Autodesk Inventor part; units mm, degrees
ref_plane "Work Plane1" through (0, 0, 2) normal (0, 0, -1) x (-1, 0, 0)
ref_plane "Work Plane2" through (0, 0, 15.2) normal (0, 0, -1) x (-1, 0, 0)
ref_plane "YZ Plane" through (0, 0, 0) normal (1, 0, 0) x (0, 1, 0)
sketch "Sketch1" plane through (0, 0, 0) normal (0, 0, 1) x (1, 0, 0)
  circle A0 centre (0, 0) radius 37.5 construction
  circle A1 centre (0, 0) radius 38.1
  line L0 (0, 0) -> (0, 82.8508) construction
  line L1 (-6, 47.5) -> (6, 47.5)
  line L2 (20, 35.8331) -> (20, 38.2923)
  line L3 (-20, 35.8331) -> (-20, 38.2923)
  arc A2 (-6, 47.5) -> (-18.8366, 41.4986) centre (-6, 30.7709) ccw
  arc A3 (18.8366, 41.4986) -> (6, 47.5) centre (6, 30.7709) ccw
  arc A4 (-18.8366, 41.4986) -> (-20, 38.2923) centre (-15, 38.2923) ccw
  arc A5 (20, 38.2923) -> (18.8366, 41.4986) centre (15, 38.2923) ccw
  arc A6 (17.1022, 34.0459) -> (-17.1022, 34.0459) centre (0, 0) ccw
  arc A7 (-20, 35.8331) -> (-17.1022, 34.0459) centre (-18, 35.8331) ccw
  arc A8 (17.1022, 34.0459) -> (20, 35.8331) centre (18, 35.8331) ccw
  point P0 (20, 32.4285)
  point P1 (20, 39.9285)
  point P2 (-20, 32.4285)
  point P3 (-20, 39.9285)
  point P4 (-17.1022, 34.0459)
  dimension "d0" = 75
  dimension "d1" = 0.6
  dimension "d22" = 12
  dimension "d23" = 6
  dimension "d24" = 47.5
  dimension "d25" = 7.5
  dimension "d26" = 7.5
  dimension "d27" = 40
  dimension "d28" = 20
  dimension "d29" = 5
  dimension "d30" = 2
extrude "Extrusion1" add sketch "Sketch1" along normal blind 30.4 contours A1 A7 L3 A4 A2 L1 A3 A5 L2 A8
sketch "Sketch2" plane through (-6, 47.5, 0) normal (0, 1, 0) x (1, 0, 0)
  line L0 (12, -30.4) -> (0, -30.4)
  line L1 (12, 0) -> (12, -30.4)
  line L2 (0, -30.4) -> (16.9706, -30.4) construction
  line L3 (12, -30.4) -> (24.8366, -30.4)
  line L4 (0, 0) -> (0, -30.4)
  line L5 (23.1022, 0) -> (-11.1022, 0)
  circle A0 centre (6, -22.4) radius 3.9
  circle A1 centre (6, -8) radius 3.9
  point P0 (6, 0)
  dimension "d34" = 7.8
  dimension "d35" = 7.8
  dimension "d38" = 12
  dimension "d39" = 6
  dimension "d40" = 6
  dimension "d41" = 8
  dimension "d42" = 8
extrude "Extrusion2" cut sketch "Sketch2" against normal blind 15 contours A0 | A1
ref_plane "Work Plane1" through (0, 0, 2) normal (0, 0, -1) x (-1, 0, 0)
sketch "Sketch3" plane through (0, 0, 2) normal (0, 0, -1) x (-1, 0, 0)
  arc A0 (17.1022, 34.0459) -> (-17.1022, 34.0459) centre (0, 0) ccw
  line L0 (-15, 35.023) -> (-15, 36.023)
  line L1 (15, 35.023) -> (15, 36.023)
  line L2 (0, 0) -> (0, 39.8883) construction
  arc A1 (15, 36.023) -> (-15, 36.023) centre (0, 0) ccw
  dimension "d44" = 1
  dimension "d45" = 30
  dimension "d46" = 15
extrude "Extrusion3" cut sketch "Sketch3" against normal blind 26.4
sketch "Sketch4" plane through (0, 0, 0) normal (0, 0, -1) x (-1, 0, 0)
  line L0 (-6, 47.5) -> (6, 47.5)
  circle A0 centre (-12, 41.5) radius 2.4
  line L1 (-6, 47.5) -> (6, 47.5)
  circle A1 centre (12, 41.5) radius 2.4
  point P0 (0, 0)
  dimension "d52" = 4.8
  dimension "d53" = 12
  dimension "d54" = 6
  dimension "d55" = 4.8
  dimension "d56" = 12
  dimension "d57" = 6
extrude "Extrusion4" cut sketch "Sketch4" against normal blind 8
ref_plane "Work Plane2" through (0, 0, 15.2) normal (0, 0, -1) x (-1, 0, 0)
mirror "Mirror1" about plane through (0, 0, 15.2) normal (0, 0, -1) of "Extrusion4"
equation "\"d23\" = 0.5 * d22"
equation "\"d35\" = d34"
equation "\"d39\" = 0.5 * d38"
equation "\"d40\" = 0.5 * d38"
equation "\"d42\" = d41"
equation "\"d46\" = 0.5 * d45"
equation "\"d57\" = d54"
properties part number "PipeHolder" material "ABS Plastic"
Can you work these out from the model? Positions are in its coordinate system, mm. A direction names the side the tool comes from. Round coordinates to 2 decimals unless told otherwise and drop trailing zeros. Loops run counter-clockwise (first coordinate to the right, second up) from the corner with the lowest first, then second, coordinate; pieces in that order, holes last. Notation, with made-up numbers: (-31, 50.5) - (-18, 50.5) arc R22 ccw to (-18, 78.5) - close; hole circle Ø6 at (19, 63.5). An arc over 180 degrees is marked (long way). Answer in a Markdown table with one row per item. Add a question column.
Q1. I need wall thicknesses on L1, parallel to X at y = 41.75, z = 24.5; L2, parallel to Z at x = 0.5, y = 38.25; L3, parallel to Y at x = 14, z = 27. Which ranges of each line are inside material? Lowest first, please.
Q2. I want a section at B-B on x = -2.5. List the corners of the cut face in (y, z) for me, and give its area (3 significant figures).
Q3. I want a section at C-C on z = 8.5. List the corners of the cut face in (x, y) for me.
Q4. I want a section at A-A on z = 3. List the corners of the cut face in (x, y) for me, and give its area (3 significant figures).
Q5. For pin 1 Ø2.5 at (x, y) = (-12, 41) entering from -Z; pin 2 Ø0.5 at (y, z) = (35.5, 16.5) entering from -X; pin 3 Ø3 at (y, z) = (44, 9) entering from +X; pin 4 Ø8 at (x, z) = (10.5, 25.5) entering from +Y, each with a flat end and sliding along its axis, tell me the tip position at first contact or that it passes through.
Q6. We'd pull the mould along Z, two halves only. Please class faces 1 (the flat face through (0, 41, 30.4)), 2 (the cylindrical face through (12.99, 45.97, 14.99)), 3 (the flat face through (0.1, 38.5, 2)): pulls with the +Z half, pulls with the -Z half, needs draft (parallel to the pull), parting line crosses it, or undercut.
Q7. I want a section at D-D on y = 45. List the corners of the cut face in (x, z) for me.
Q8. Which directions (+Z, -Z, +X, -X, +Y, -Y) give clear straight access to the entire face, cutting with the end or side of a thin tool? Please do faces 4 (the flat face through (20, 37, 15)), 5 (the flat face through (12, 42, 8)), 6 (the cylindrical face through (-19.7, 40, 15)), 7 (the cylindrical face through (12.52, 43.843, 26.456)), 8 (the cylindrical face through (-0.22, 39.02, 15.02)).
A:
| question | item | result |
|---|---|---|
| 1 | L1 | -18.62 to -14.39, -9.61 to -3.29, 3.29 to 9.61, 14.39 to 18.62 |
| 1 | L2 | 0 to 2, 28.4 to 30.4 |
| 1 | L3 | 36.42 to 40.17, 42.83 to 45.46 |
| 2 | outline | (38.02, 0) - (47.5, 0) - (47.5, 5.01) - (38.94, 5.01) - (38.94, 2) - (38.02, 2) - close; (38.02, 28.4) - (38.94, 28.4) - (38.94, 25.39) - (47.5, 25.39) - (47.5, 30.4) - (38.02, 30.4) - close; (38.94, 10.99) - (47.5, 10.99) - (47.5, 19.41) - (38.94, 19.41) - close |
| 2 | area | 161 mm^2 |
| 3 | outline | (-20, 35.83) arc R2 ccw to (-17.1, 34.05) arc R38.1 cw to (-15, 35.02) - (-15, 36.02) arc R39.02 cw to (-3.87, 38.83) - (-3.87, 47.5) - (-6, 47.5) arc R16.73 ccw to (-18.84, 41.5) arc R5 ccw to (-20, 38.29) - close; (3.87, 38.83) arc R39.02 cw to (15, 36.02) - (15, 35.02) arc R38.1 cw to (17.1, 34.05) arc R2 ccw to (20, 35.83) - (20, 38.29) arc R5 ccw to (18.84, 41.5) arc R16.73 ccw to (6, 47.5) - (3.87, 47.5) - close |
| 4 | outline | (-20, 35.83) arc R2 ccw to (-17.1, 34.05) arc R38.1 cw to (-15, 35.02) - (-15, 36.02) arc R39.02 cw to (15, 36.02) - (15, 35.02) arc R38.1 cw to (17.1, 34.05) arc R2 ccw to (20, 35.83) - (20, 38.29) arc R5 ccw to (18.84, 41.5) arc R16.73 ccw to (6, 47.5) - (-6, 47.5) arc R16.73 ccw to (-18.84, 41.5) arc R5 ccw to (-20, 38.29) - close; hole circle Ø4.8 at (-12, 41.5); hole circle Ø4.8 at (12, 41.5) |
| 4 | area | 316 mm^2 |
| 5 | pin 1 | z = 8 |
| 5 | pin 2 | x = -20 |
| 5 | pin 3 | x = 17.93 |
| 5 | pin 4 | y = 47.49 |
| 6 | face 1 | pulls with the +Z half |
| 6 | face 2 | needs draft |
| 6 | face 3 | undercut |
| 7 | outline | (-14.8, 0) - (14.8, 0) - (14.8, 30.4) - (-14.8, 30.4) - close; hole circle Ø7.8 at (0, 8); hole circle Ø7.8 at (0, 22.4) |
| 8 | face 4 | +Z, -Z, +X, +Y, -Y |
| 8 | face 5 | -Z |
| 8 | face 6 | +Z, -Z, -X, +Y |
| 8 | face 7 | +Z |
| 8 | face 8 | -Y |
